from build123d import *

# Parameters (mm, degrees)
SKETCH1_W           = 23.5
SKETCH1_H           = 90
BOSS_EXTRUDE1_DEPTH = 1.5875
BOSS_EXTRUDE2_DEPTH = 1.5875
CUT_EXTRUDE3_DEPTH  = 2.5875
LPATTERN1_COUNT     = 3
LPATTERN1_PITCH     = 30
SKETCH5_R           = 2.286
CUT_EXTRUDE4_DEPTH  = 2.5875
CHAMFER1_SIZE       = 2
SKETCH6_W           = 3.25
SKETCH6_H           = 6
BOSS_EXTRUDE3_DEPTH = 1.5875
FILLET1_R           = 1
FILLET2_R           = 0.5
SKETCH7_R           = 0.75
CUT_EXTRUDE5_DEPTH  = 2.5875


with BuildPart() as part:
    # Sketch1 → Boss-Extrude1 (new body)
    with BuildSketch(Plane(origin=(0, 0, 0), x_dir=(1, 0, 0), z_dir=(0, 1, 0))):
        Rectangle(SKETCH1_W, SKETCH1_H)
    extrude(amount=BOSS_EXTRUDE1_DEPTH)

    # Sketch2 → Boss-Extrude2 (add)
    with BuildSketch(Plane(origin=(0, 1.5875, 0), x_dir=(1, 0, 0), z_dir=(0, 1, 0))):
        with BuildLine():
            Line((11.75, -29.5), (12.590477082, -26.25290926))
            ThreePointArc((12.590477082, -26.25290926), (3.882734587, -21.830732226), (9.929449472, -29.5))
            Line((9.929449472, -29.5), (11.75, -29.5))
        make_face()
    boss_extrude2 = extrude(amount=-BOSS_EXTRUDE2_DEPTH)

    # Sketch4 → Cut-Extrude3 (cut, through all)
    with BuildSketch(Plane(origin=(0, 1.5875, 0), x_dir=(1, 0, 0), z_dir=(0, 1, 0))):
        with BuildLine():
            Line((10.75, -21), (9.75, -21))
            Line((9.75, -21), (9.75, -37))
            ThreePointArc((9.75, -37), (9.503785707, -37.249971335), (9.250114653, -37.007570546))
            Line((9.250114653, -37.007570546), (8.75, -20.5))
            Line((8.75, -20.5), (10.15, -20.5))
            ThreePointArc((10.15, -20.5), (11.018993513, -21.085452592), (11.75, -21.836141596))
            Line((11.75, -21.836141596), (11.75, -22))
            ThreePointArc((11.75, -22), (11.285533906, -21.464466094), (10.75, -21))
        make_face()
    cut_extrude3 = extrude(amount=-CUT_EXTRUDE3_DEPTH, mode=Mode.SUBTRACT)

    # LPattern1: Boss-Extrude2, Cut-Extrude3 ×3
    with Locations(*[(0, 0, -i * LPATTERN1_PITCH) for i in range(1, LPATTERN1_COUNT)]):
        add(boss_extrude2)
        add(cut_extrude3, mode=Mode.SUBTRACT)

    # Sketch5 → Cut-Extrude4 (cut, through all)
    with BuildSketch(Plane(origin=(0, 1.5875, 0), x_dir=(1, 0, 0), z_dir=(0, 1, 0))):
        with Locations((-8, -31)):
            Circle(SKETCH5_R)
        with Locations((8, -15)):
            Circle(SKETCH5_R)
        with Locations((-8, 31)):
            Circle(SKETCH5_R)
        with Locations((8, 15)):
            Circle(SKETCH5_R)
        with Locations((-8, 0)):
            Circle(SKETCH5_R)
    extrude(amount=-CUT_EXTRUDE4_DEPTH, mode=Mode.SUBTRACT)

    # Chamfer1
    chamfer1_edges = [part.edges().sort_by_distance(p)[0] for p in [
        (11.75, 0.79375, 45),
        (-11.75, 0.79375, 45),
    ]]
    chamfer(chamfer1_edges, length=CHAMFER1_SIZE)

    # Sketch6 → Boss-Extrude3 (add)
    with BuildSketch(Plane(origin=(0, 1.5875, 0), x_dir=(1, 0, 0), z_dir=(0, 1, 0))):
        with Locations((-13.375, 42)):
            Rectangle(SKETCH6_W, SKETCH6_H)
        with Locations((13.375, 42)):
            Rectangle(SKETCH6_W, SKETCH6_H)
    extrude(amount=-BOSS_EXTRUDE3_DEPTH)

    # Fillet1
    fillet1_edges = [part.edges().sort_by_distance(p)[0] for p in [
        (8.75, 0.79375, -39.5),
        (8.75, 0.79375, 20.5),
        (8.75, 0.79375, -9.5),
    ]]
    fillet(fillet1_edges, radius=FILLET1_R)

    # Fillet2
    fillet2_edges = [part.edges().sort_by_distance(p)[0] for p in [
        (9.75, 0.79375, -39),
        (9.75, 0.79375, 21),
        (9.75, 0.79375, -9),
    ]]
    fillet(fillet2_edges, radius=FILLET2_R)

    # Sketch7 → Cut-Extrude5 (cut, through all)
    with BuildSketch(Plane(origin=(0, 1.5875, 0), x_dir=(1, 0, 0), z_dir=(0, 1, 0))):
        with Locations((-11.75, 38.25)):
            Circle(SKETCH7_R)
    extrude(amount=-CUT_EXTRUDE5_DEPTH, mode=Mode.SUBTRACT)


solid = part.part
Part model, mm, in its own coordinate system. A direction names the side the tool comes from. Coordinates: 2 decimals unless noted, no trailing zeros. Loops run counter-clockwise (first coordinate to the right, second up) from the corner with the lowest first, then second, coordinate; pieces in that order, holes last. Notation, with made-up numbers: M -36.5,22 L -31.5,22 A19 cw -31.5,26 Z; hole C 78,34.25 d2. An arc over 180 degrees is marked long. Use a Markdown table: item, result. Add a question column.
Q1. Cut at B-B (z = 15). Write the cut outline in (x, y), and give its area (3 significant figures).
Q2. Which spindle directions (+Z, -Z, +X, -X, +Y, -Y) get a long thin tool onto all of the face, cutting with end or side? Do faces 5 (the flat face through (0, 1, -45)), 6 (the flat face through (-11.75, 1, 3)), 7 (the flat face through (12.164, 0.805, -2.101)). Say none if no direction does.
Q3. Cut at A-A (x = -8). Write the cut outline in (y, z).
Q4. Pin check, flat tips, straight feed: P1, Ø0.5, axis at y = 1, z = 15.5, coming from the +X side; P2, Ø0.5, axis at x = -13, y = 1, coming from the +Z side; P3, Ø1.5, axis at x = -3.5, z = 8.5, coming from the -Y side. Stop position of each tip, or through.
Q5. Cut at D-D (y = 0.6). Give the number of separate pieces and of enclosed holes in the cut face, and give its area (3 significant figures).
Q6. Mould opens along Z. For faces 1 (the cylindrical face through (-8.298, 0.805, 28.733)), 2 (the flat face through (12.164, 0.805, 27.899)), 3 (the flat face through (13, 1, -39)), 4 (the flat face through (11.75, 1, 36)) say: +Z half, -Z half, draft (parallel to the pull), parting line (faces both ways), or undercut.
Q7. Probe L1, parallel to Z at x = 8, y = 0.8; L2, parallel to X at y = 1, z = -15; L3, parallel to Z at x = 7.25, y = 0.2. List the from-to ranges inside material, lowest first.
Q8. Cut at C-C (x = 8). Write the cut outline in (y, z).
Worked out:
| question | item | result |
|---|---|---|
| 1 | outline | M -11.75,0 L 5.71,0 L 5.71,1.59 L -11.75,1.59 Z; M 10.29,0 L 11.75,0 L 11.75,1.59 L 10.29,1.59 Z |
| 1 | area | 30.0 mm2 |
| 2 | face 5 | -Z, +X, -X, +Y, -Y |
| 2 | face 6 | +Z, -X, +Y, -Y |
| 2 | face 7 | +X, +Y, -Y |
| 3 | outline | M 0,-45 L 1.59,-45 L 1.59,-33.29 L 0,-33.29 Z; M 0,-28.71 L 1.59,-28.71 L 1.59,-2.29 L 0,-2.29 Z; M 0,2.29 L 1.59,2.29 L 1.59,28.71 L 0,28.71 Z; M 0,33.29 L 1.59,33.29 L 1.59,45 L 0,45 Z |
| 4 | P1 | stops at x = 11.75 |
| 4 | P2 | stops at z = -39 |
| 4 | P3 | stops at y = 0 |
| 5 | separate pieces | 1 |
| 5 | enclosed holes | 5 |
| 5 | area | 2,040 mm2 |
| 6 | face 1 | undercut |
| 6 | face 2 | +Z half |
| 6 | face 3 | undercut |
| 6 | face 4 | draft |
| 7 | L1 | z = -45 to -17.29, -12.71 to 12.71, 17.29 to 45 |
| 7 | L2 | x = -11.75 to 5.71, 10.29 to 11.75 |
| 7 | L3 | z = -45 to -17.16, -12.84 to 12.84, 17.16 to 45 |
| 8 | outline | M 0,-45 L 1.59,-45 L 1.59,-17.29 L 0,-17.29 Z; M 0,-12.71 L 1.59,-12.71 L 1.59,12.71 L 0,12.71 Z; M 0,17.29 L 1.59,17.29 L 1.59,45 L 0,45 Z |
